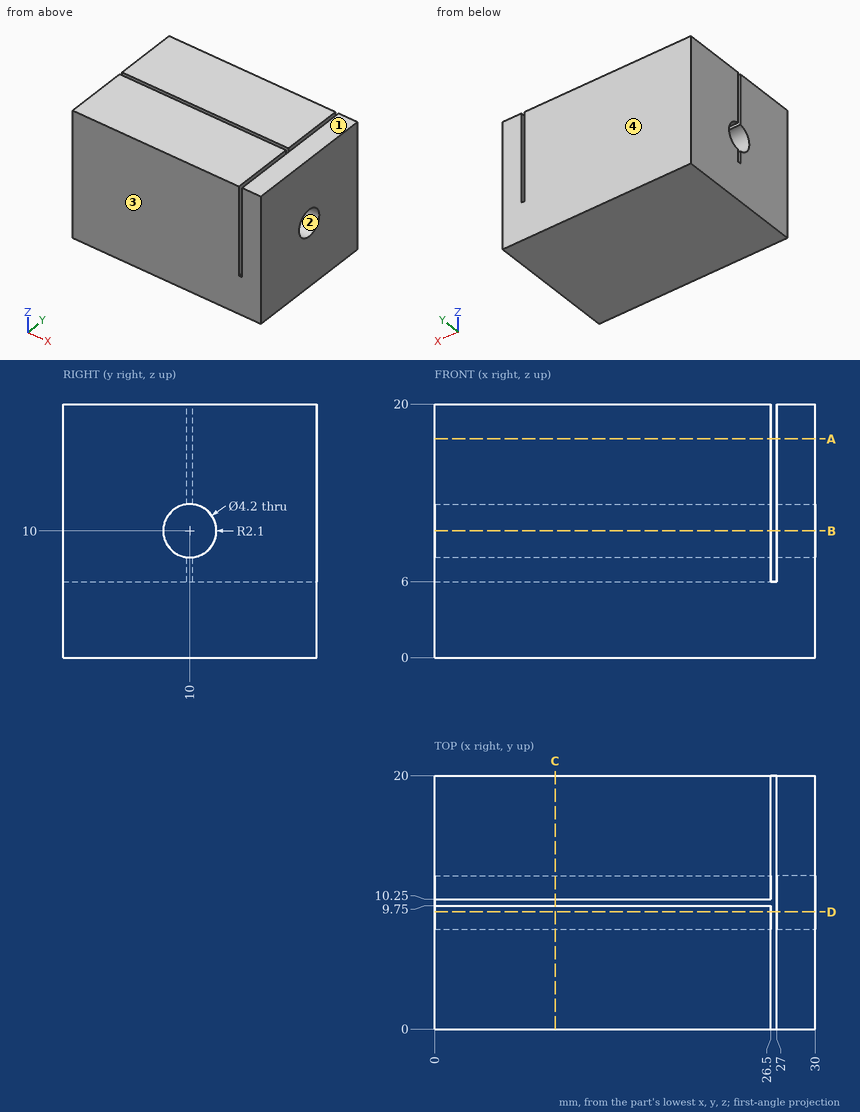
Design review of the part shown in the three views and the two pictorial views. Dimensions are in mm from the part's minimum x, y and z. Coordinates: 2 decimals unless noted, no trailing zeros. Order: outer loops, then holes, each group sorted by start corner. A loop starts at its lowest first (then second) coordinate and runs counter-clockwise, first axis right, second up. Notation, with made-up numbers: (24.25, 36.25) -> (38.25, 36.25) arc R21 ccw to (38.25, 66.25) -> close; hole circle Ø1 at (56.5, 84). An arc over 180 degrees is marked (long way). Use one line per item in the form item = value. Start each with the question number.
(1) The part is to be moulded in two halves that separate along Y. For the marked faces 1, 2, 3 and 4, say which applies: +Y half, -Y half, draft (parallel to the pull), parting line (faces both ways), or undercut.
(2) Add section D-D on y = 9.25. State the section outline as (x, z) points.
(3) Add section A-A on z = 17.25. State the section outline as (x, y) points, plus the area to 3 significant figures.
(4) Insertion check: pin 1 (3.5 mm diameter, centred on y = 10, z = 10, fed in from +X). The pin has a flat end and moves straight along its axis. Give the tip position at first contact, or say it passes through.
(5) Add section C-C on x = 9.5. State the section outline as (y, z) points, plus the area to 3 significant figures.
(6) For probe 1 along Y at (x, z) = (13.5, 14); probe 2 along X at (y, z) = (1, 16); probe 3 along Z at (x, y) = (28.1, 10), list the stretches that pass through material, from the lowest coordinate up.
(7) Add section B-B on z = 10. State the section outline as (x, y) points.
Answer block:
q1.face_1 = draft
q1.face_2 = undercut
q1.face_3 = -Y half
q1.face_4 = +Y half
q2.outline = (0, 0) -> (30, 0) -> (30, 8.04) -> (27, 8.04) -> (27, 6) -> (26.5, 6) -> (26.5, 8.04) -> (0, 8.04) -> close; (0, 11.96) -> (26.5, 11.96) -> (26.5, 20) -> (0, 20) -> close; (27, 11.96) -> (30, 11.96) -> (30, 20) -> (27, 20) -> close
q3.outline = (0, 0) -> (26.5, 0) -> (26.5, 9.75) -> (0, 9.75) -> close; (0, 10.25) -> (26.5, 10.25) -> (26.5, 20) -> (0, 20) -> close; (27, 0) -> (30, 0) -> (30, 20) -> (27, 20) -> close
q3.area = 577 mm²
q4.pin_1 = through
q5.outline = (0, 0) -> (20, 0) -> (20, 20) -> (10.25, 20) -> (10.25, 12.09) arc R2.1 cw to (10.25, 7.91) -> (10.25, 6) -> (9.75, 6) -> (9.75, 7.91) arc R2.1 cw to (9.75, 12.09) -> (9.75, 20) -> (0, 20) -> close
q5.area = 381 mm²
q6.probe_1 = 0 to 9.75, 10.25 to 20
q6.probe_2 = 0 to 26.5, 27 to 30
q6.probe_3 = 0 to 7.9, 12.1 to 20
q7.outline = (0, 0) -> (26.5, 0) -> (26.5, 7.9) -> (0, 7.9) -> close; (0, 12.1) -> (26.5, 12.1) -> (26.5, 20) -> (0, 20) -> close; (27, 0) -> (30, 0) -> (30, 7.9) -> (27, 7.9) -> close; (27, 12.1) -> (30, 12.1) -> (30, 20) -> (27, 20) -> close
